Read the model definition and answer for the solid it produces. Units are mm, in the model's axes. Coordinates: 2 decimals unless noted, no trailing zeros. Write each loop counter-clockwise with the first axis right and the second up, starting at its lowest first coordinate (ties: lowest second). Pieces come first, ordered by that corner, then holes. Notation, with made-up numbers: (41, -10) -> (56, -10) arc R17 cw to (56, 22) -> close; hole circle Ø8 at (81.5, 36.5). An arc over 180 degrees is marked (long way). One line per item, written item: value. Start each with the question number.
from build123d import *

# Parameters (mm, degrees)
F0_R     = 3.175
F1_DEPTH = 31.75


with BuildPart() as f1:
    # F0 (on Front) → F1 (new body)
    with BuildSketch(Plane.XZ):
        with BuildLine():
            Line((22.0577025061, 15.4224140263), (15.7504882737, 65.484375))
            ThreePointArc((15.7504882737, 65.484375), (15.8438414904, 64.4941387366), (15.875, 63.5))
            ThreePointArc((15.875, 63.5), (11.2253201513, 52.2746798487), (0, 47.625))
            Line((0, 47.625), (0, 9.525))
            ThreePointArc((0, 9.525), (6.7351920908, 6.7351920908), (9.525, 0))
            Line((9.525, 0), (36.5125, 0))
            ThreePointArc((36.5125, 0), (38.9384772185, 5.7120069047), (44.7334821429, 7.9324362036))
            Line((44.7334821429, 7.9324362036), (29.6616113193, 8.4710609247))
            ThreePointArc((29.6616113193, 8.4710609247), (24.5813298898, 10.5484079743), (22.0577025061, 15.4224140263))
        make_face()
        with BuildLine():
            ThreePointArc((9.4502929642, 115.490625), (9.5063048942, 114.896483242), (9.525, 114.3))
            ThreePointArc((9.525, 114.3), (6.7351920908, 107.5648079092), (0, 104.775))
            Line((0, 104.775), (0, 100.0252))
            Line((0, 100.0252), (0, 79.375))
            ThreePointArc((0, 79.375), (10.5003255158, 75.40625), (15.7504882737, 65.484375))
            Line((15.7504882737, 65.484375), (9.4502929642, 115.490625))
        make_face()
        with BuildLine():
            Line((0, 100.0252), (0, 104.775))
            ThreePointArc((0, 104.775), (-7.14375, 107.9998046905), (-9.4502929642, 115.490625))
            Line((-9.4502929642, 115.490625), (-15.7504882737, 65.484375))
            ThreePointArc((-15.7504882737, 65.484375), (-10.5003255158, 75.40625), (0, 79.375))
            Line((0, 79.375), (0, 100.0252))
        make_face()
        with Locations((-3.175, 100.0252)):
            Circle(F0_R, mode=Mode.SUBTRACT)
        with BuildLine():
            ThreePointArc((0, 104.775), (6.7351920908, 107.5648079092), (9.525, 114.3))
            ThreePointArc((9.525, 114.3), (9.5063048942, 114.896483242), (9.4502929642, 115.490625))
            ThreePointArc((9.4502929642, 115.490625), (0, 123.825), (-9.4502929642, 115.490625))
            ThreePointArc((-9.4502929642, 115.490625), (-7.14375, 107.9998046905), (0, 104.775))
        make_face()
        with BuildLine():
            ThreePointArc((3.175, 114.3), (2.2450640303, 112.0549359697), (0, 111.125))
            ThreePointArc((0, 111.125), (-2.2450640303, 116.5450640303), (3.175, 114.3))
        make_face(mode=Mode.SUBTRACT)
        with BuildLine():
            Line((36.5125, 0), (9.525, 0))
            ThreePointArc((9.525, 0), (6.9705567315, -6.4912990883), (0.6773435479, -9.500885786))
            Line((0.6773435479, -9.500885786), (44.7324052746, -7.9324746146))
            ThreePointArc((44.7324052746, -7.9324746146), (38.9380895153, -5.7116327839), (36.5125, 0))
        make_face()
        with BuildLine():
            ThreePointArc((0, 9.525), (-7.063929059, 6.3895642457), (-9.4772553384, -0.9525))
            ThreePointArc((-9.4772553384, -0.9525), (-6.3895642457, -7.063929059), (0, -9.525))
            Line((0, -9.525), (0.6773435479, -9.500885786))
            ThreePointArc((0.6773435479, -9.500885786), (6.9705567315, -6.4912990883), (9.525, 0))
            Line((9.525, 0), (3.175, 0))
            ThreePointArc((3.175, 0), (-2.2450640303, -2.2450640303), (0, 3.175))
            Line((0, 3.175), (0, 9.525))
        make_face()
        with BuildLine():
            ThreePointArc((9.525, 0), (6.7351920908, 6.7351920908), (0, 9.525))
            Line((0, 9.525), (0, 3.175))
            ThreePointArc((0, 3.175), (2.2450640303, 2.2450640303), (3.175, 0))
            Line((3.175, 0), (9.525, 0))
        make_face()
        with BuildLine():
            ThreePointArc((52.3875, 0), (50.1620069047, 5.5115227815), (44.7334821429, 7.9324362036))
            ThreePointArc((44.7334821429, 7.9324362036), (38.9384772185, 5.7120069047), (36.5125, 0))
            ThreePointArc((36.5125, 0), (38.9380895153, -5.7116327839), (44.7324052746, -7.9324746146))
            ThreePointArc((44.7324052746, -7.9324746146), (50.1616327839, -5.5119104847), (52.3875, 0))
        make_face()
        with BuildLine():
            ThreePointArc((47.625, 0), (44.45, -3.175), (41.275, 0))
            ThreePointArc((41.275, 0), (44.45, 3.175), (47.625, 0))
        make_face(mode=Mode.SUBTRACT)
        with BuildLine():
            ThreePointArc((0, 79.375), (-10.5003255158, 75.40625), (-15.7504882737, 65.484375))
            ThreePointArc((-15.7504882737, 65.484375), (-15.8737438155, 63.6997054867), (-15.7954255641, 61.9125))
            ThreePointArc((-15.7954255641, 61.9125), (-10.6492737428, 51.7267849017), (0, 47.625))
            Line((0, 47.625), (0, 60.325))
            ThreePointArc((0, 60.325), (-3.175, 63.5), (0, 66.675))
            Line((0, 66.675), (0, 79.375))
        make_face()
        with BuildLine():
            ThreePointArc((15.875, 63.5), (15.8438414904, 64.4941387366), (15.7504882737, 65.484375))
            ThreePointArc((15.7504882737, 65.484375), (10.5003255158, 75.40625), (0, 79.375))
            Line((0, 79.375), (0, 66.675))
            ThreePointArc((0, 66.675), (2.2450640303, 65.7450640303), (3.175, 63.5))
            ThreePointArc((3.175, 63.5), (2.2450640303, 61.2549359697), (0, 60.325))
            Line((0, 60.325), (0, 47.625))
            ThreePointArc((0, 47.625), (11.2253201513, 52.2746798487), (15.875, 63.5))
        make_face()
        with BuildLine():
            ThreePointArc((0, 47.625), (-10.6492737428, 51.7267849017), (-15.7954255641, 61.9125))
            Line((-15.7954255641, 61.9125), (-9.4772553384, -0.9525))
            ThreePointArc((-9.4772553384, -0.9525), (-7.063929059, 6.3895642457), (0, 9.525))
            Line((0, 9.525), (0, 47.625))
        make_face()
    extrude(amount=F1_DEPTH)


solid = f1.part
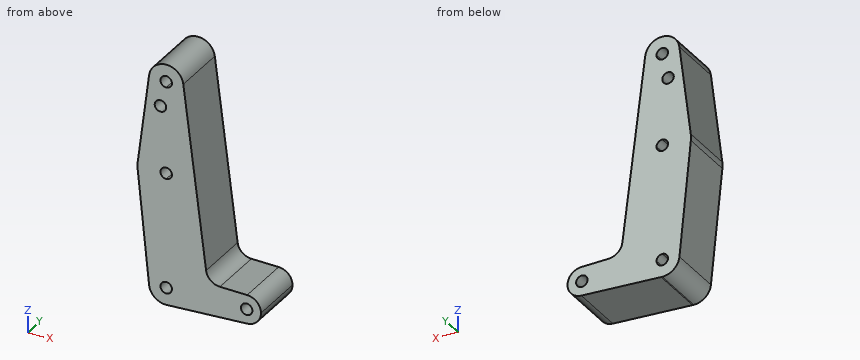
1. Find the intervals of material crossed by probe 1 along Z at (x, y) = (1.5, -13.5); probe 2 along Z at (x, y) = (44.45, -12) (3 decimals); probe 3 along Z at (x, y) = (-2, -30), in increasing order. Write a range as from..to.
2. Given pin 1 (5.5 mm diameter, centred on x = -3.18, z = 100.03, fed in from +Y); pin 2 (1 mm diameter, centred on x = 18, y = -20, fed in from -Z); pin 3 (5 mm diameter, centred on y = -18.5, z = 23.5, fed in from -X); pin 4 (12 mm diameter, centred on y = -18, z = 25.5, fed in from -X), each flat-ended and moving along its own axis, determine where each tip first touches the part or whether it passes through.
3. A cutting plane is placed at A-A on y = -3.5. Count the separate pieces of the cut face and the enclosed holes in it, then the cut area to 3 significant figures.
4. A cutting plane is placed at C-C on x = 8. Give the vertices of the cut face in (y, z), then the cut area to 3 significant figures.
5. A cutting plane is placed at B-B on x = 20. Give the vertices of the cut face in (y, z), then the cut area to 3 significant figures.
Derived:
1. probe 1: z = -9.47..-2.8, 2.8..60.7, 66.3..111.5, 117.1..123.71
1. probe 2: z = -7.943..-3.175, 3.175..7.943
1. probe 3: z = -9.31..-2.47, 2.47..61.03, 65.97..97.08, 102.97..111.83, 116.77..123.61
2. pin 1: passes through
2. pin 2: stops at z = -8.9
2. pin 3: stops at x = -12.19
2. pin 4: stops at x = -12.74
3. separate pieces: 1
3. enclosed holes: 5
3. area: 4,110 mm2
4. outline: (-31.75, -9.24) -> (0, -9.24) -> (0, 119.47) -> (-31.75, 119.47) -> close
4. area: 4,090 mm2
5. outline: (-31.75, -8.81) -> (0, -8.81) -> (0, 31.75) -> (-31.75, 31.75) -> close
5. area: 1,290 mm2
